from build123d import *

# Parameters (mm, degrees)
SKETCH2_W           = 20
SKETCH2_H           = 20
BOSS_EXTRUDE1_DEPTH = 700
SKETCH3_W           = 19
SKETCH3_H           = 19
CUT_EXTRUDE1_DEPTH  = 700
SKETCH5_R           = 2.5
CUT_EXTRUDE2_DEPTH  = 20
SKETCH6_R           = 4
CUT_EXTRUDE3_DEPTH  = 20
SKETCH7_R           = 2.5
CUT_EXTRUDE4_DEPTH  = 20


with BuildPart() as part:
    # Sketch2 → Boss-Extrude1 (new body)
    with BuildSketch(Plane.XY):
        Rectangle(SKETCH2_W, SKETCH2_H)
    extrude(amount=BOSS_EXTRUDE1_DEPTH)

    # Sketch3 → Cut-Extrude1 (cut)
    with BuildSketch(Plane(origin=(0, 0, 0), x_dir=(-1, 0, 0), z_dir=(0, 0, -1))):
        Rectangle(SKETCH3_W, SKETCH3_H)
    extrude(amount=-CUT_EXTRUDE1_DEPTH, mode=Mode.SUBTRACT)

    # Sketch5 → Cut-Extrude2 (cut)
    with BuildSketch(Plane.XZ.offset(10)):
        with Locations(Location((0, 635, 0), (0, 0, 270))):
            Circle(SKETCH5_R)
        with Locations(Location((0, 675, 0), (0, 0, 270))):
            Circle(SKETCH5_R)
    extrude(amount=-CUT_EXTRUDE2_DEPTH, mode=Mode.SUBTRACT)

    # Sketch6 → Cut-Extrude3 (cut)
    with BuildSketch(Plane(origin=(10, 0, 0), x_dir=(0, 0, -1), z_dir=(1, 0, 0))):
        with Locations(Location((-270, 0, 0), (0, 0, 90))):
            Circle(SKETCH6_R)
    extrude(amount=-CUT_EXTRUDE3_DEPTH, mode=Mode.SUBTRACT)

    # Sketch7 → Cut-Extrude4 (cut)
    with BuildSketch(Plane.XZ.offset(10)):
        with Locations(Location((0, 20, 0), (0, 0, 270))):
            Circle(SKETCH7_R)
        with Locations(Location((0, 50, 0), (0, 0, 270))):
            Circle(SKETCH7_R)
    extrude(amount=-CUT_EXTRUDE4_DEPTH, mode=Mode.SUBTRACT)


solid = part.part
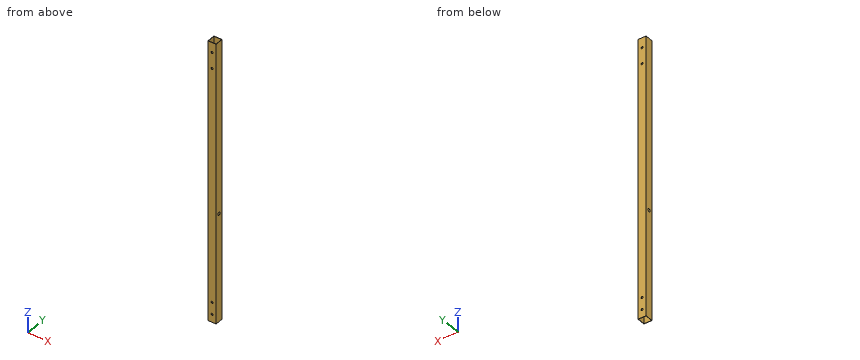
Build history of the part. All positions in model axes, mm. Give positions to 0.01 mm unless a question says otherwise; leave off trailing zeros. Loops run counter-clockwise (first coordinate to the right, second up) from the corner with the lowest first, then second, coordinate; pieces in that order, holes last. Notation, with made-up numbers: (82.25, -11.5) -> (119.25, -11.5) arc R14 ccw to (119.25, 15.5) -> close; hole circle Ø10 at (-23, 17.5). An arc over 180 degrees is marked (long way). Answer in a Markdown table with one row per item.
Item 1: Slice it at A-A on y = 0. Write the cut outline in (x, z).
Findings below:
| item | result |
|---|---|
| outline | (-10, 0) -> (-9.5, 0) -> (-9.5, 266) -> (-10, 266) -> close; (-10, 274) -> (-9.5, 274) -> (-9.5, 700) -> (-10, 700) -> close; (9.5, 0) -> (10, 0) -> (10, 266) -> (9.5, 266) -> close; (9.5, 274) -> (10, 274) -> (10, 700) -> (9.5, 700) -> close |
Item 2: Slice it at B-B on z = 556.5. Write the cut outline in (x, y), plus the area to 3 significant figures.
Findings below:
| item | result |
|---|---|
| outline | (-10, -10) -> (10, -10) -> (10, 10) -> (-10, 10) -> close; hole (-9.5, -9.5) -> (9.5, -9.5) -> (9.5, 9.5) -> (-9.5, 9.5) -> close |
| area | 39.0 mm² |
Item 3: Probe line 1 along Y through (x, z) = (-4, 449); line 2 along Z through (x, y) = (-9.8, 0). List the from-to ranges inside material, lowest first. Write a range as [from, to].
Findings below:
| item | result |
|---|---|
| line 1 | y = [-10, -9.5], [9.5, 10] |
| line 2 | z = [0, 266], [274, 700] |
